Study the drawing (mm; zero at the part's minimum x, y, z) and answer. A direction names the side the tool comes from. Coordinates: 2 decimals unless noted, no trailing zeros. Order: outer loops, then holes, each group sorted by start corner. A loop starts at its lowest first (then second) coordinate and runs counter-clockwise, first axis right, second up. Notation, with made-up numbers: (26.25, -10) -> (40.25, -10) arc R30 cw to (40.25, 14) -> close; hole circle Ø7 at (23, 38). An arc over 180 degrees is marked (long way). Answer as CSV lines item,"result". Start each with the question number.
Item 1: This flat-tipped pin is pushed along its axis until it touches: pin 1 Ø2 at (x, z) = (45, 28.5) entering from +Y. Where does it stop, or does it pass through?
Item 2: Section A-A (z = 61.5) is taken. Write down the section's boundary in (x, y).
Item 3: Section C-C (x = 167) is taken. Write down the section's boundary in (y, z).
Item 4: Straight lines are drawn through the part: L1, parallel to X at y = 30, z = 9; L2, parallel to Y at x = 92.5, z = 109.8; L3, parallel to Z at x = 36.5, y = 25. For each, find the intervals that lie inside material, in ascending order.
Item 5: Section B-B (y = 42.5) is taken. Write down the section's boundary in (x, z).
Item 6: For a pull along X with two mould halves and no side action, classify the marked faces 3, 4, 5 and 6 as pulls with the +X half, pulls with the -X half, needs draft (parallel to the pull), parting line crosses it, or undercut.
Item 7: Which of the six approach directions +Z, -Z, +X, -X, +Y, -Y give full straight-line access (tool end or side, diameter ignored) to the marked faces 1 and 2?
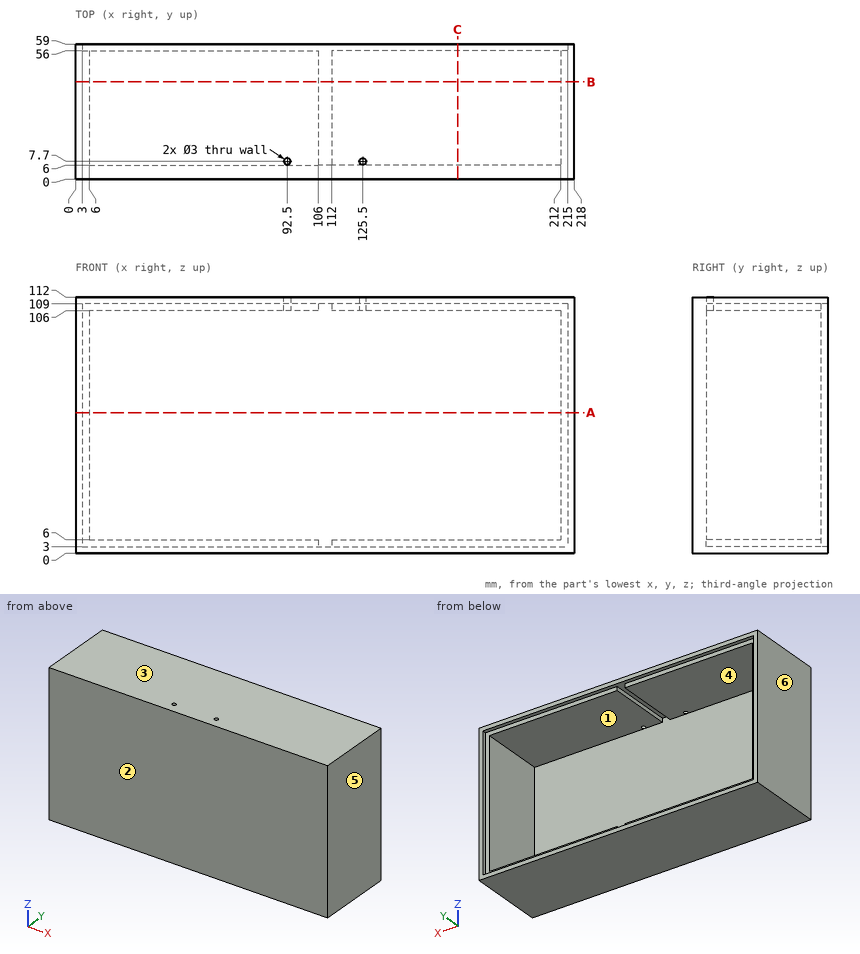
Checked values:
1,pin 1,"stops at y = 6"
2,outline,"(0, 0) -> (218, 0) -> (218, 59) -> (215, 59) -> (215, 56) -> (212, 56) -> (212, 6) -> (6, 6) -> (6, 56) -> (3, 56) -> (3, 59) -> (0, 59) -> close"
3,outline,"(0, 0) -> (59, 0) -> (59, 3) -> (56, 3) -> (56, 6) -> (6, 6) -> (6, 106) -> (56, 106) -> (56, 109) -> (59, 109) -> (59, 112) -> (0, 112) -> close"
4,L1,"x = 0 to 6, 212 to 218"
4,L2,"y = 0 to 6.2, 9.2 to 59"
4,L3,"z = 0 to 6, 106 to 112"
5,outline,"(0, 0) -> (218, 0) -> (218, 112) -> (0, 112) -> close; hole (6, 6) -> (106, 6) -> (106, 3) -> (112, 3) -> (112, 6) -> (212, 6) -> (212, 106) -> (112, 106) -> (112, 109) -> (106, 109) -> (106, 106) -> (6, 106) -> close"
6,face 3,"needs draft"
6,face 4,"undercut"
6,face 5,"pulls with the +X half"
6,face 6,"pulls with the -X half"
7,face 1,"+Y"
7,face 2,"+Z, -Z, +X, -X, -Y"
